```python
from build123d import *

# Parameters (mm, degrees)
SKETCH_W         = 45.6
SKETCH_H         = 44
SKETCH_R         = 2
PAD_DEPTH        = 3.5
PAD001_DEPTH     = 20
SKETCH002_W      = 3
SKETCH002_H      = 5
PAD002_DEPTH     = 1
CHAMFER_SIZE     = 1
CHAMFER001_ANGLE = 45
CHAMFER001_SIZE  = 2.5


with BuildPart() as part:
    # Sketch → Pad (new body)
    with BuildSketch(Plane.XY):
        Rectangle(SKETCH_W, SKETCH_H)
        with Locations((-11.4, 0)):
            Circle(SKETCH_R, mode=Mode.SUBTRACT)
        with Locations((11.4, 0)):
            Circle(SKETCH_R, mode=Mode.SUBTRACT)
    extrude(amount=PAD_DEPTH)

    # Sketch001 (on Face8 of Pad) → Pad001 (join)
    with BuildSketch(Plane.XY.offset(3.5)):
        Polygon((-22.8, 22), (-22.8, -22), (22.8, -22), (22.8, 22), (21.3, 22), (21.3, -20.5), (-21.3, -20.5), (-21.3, 22), align=None)
    extrude(amount=PAD001_DEPTH)

    # Sketch002 (on Face14 of Pad001) → Pad002 (join)
    with BuildSketch(Plane.XY.offset(23.5)):
        with Locations((-21.3, 19.5)):
            Rectangle(SKETCH002_W, SKETCH002_H)
        with Locations((21.3, 19.5)):
            Rectangle(SKETCH002_W, SKETCH002_H)
        with Locations((-21.3, -16.5)):
            Rectangle(SKETCH002_W, SKETCH002_H)
        with Locations((21.3, -16.5)):
            Rectangle(SKETCH002_W, SKETCH002_H)
    extrude(amount=PAD002_DEPTH)

    # Chamfer
    chamfer_edges = [part.edges().sort_by_distance(p)[0] for p in [
        (-21.3, -16.5, 23.5),
        (-21.3, 19.5, 23.5),
        (21.3, -16.5, 23.5),
        (21.3, 19.5, 23.5),
    ]]
    chamfer(chamfer_edges, length=CHAMFER_SIZE)

    # Chamfer001
    chamfer001_edges = [part.edges().sort_by_distance(p)[0] for p in [
        (9.4, 0, 3.5),
        (-13.4, 0, 3.5),
    ]]
    chamfer001_side = part.faces().sort_by_distance((0, 0.760558, 3.5))[0]
    chamfer(chamfer001_edges, length=CHAMFER001_SIZE, angle=CHAMFER001_ANGLE, reference=chamfer001_side)


solid = part.part
```
CAD build for the part. Positions are in the model's coordinates, mm. A direction names the side the tool comes from. Round coordinates to 2 decimals unless told otherwise and drop trailing zeros. Order: outer loops, then holes, each group sorted by start corner. A loop starts at its lowest first (then second) coordinate and runs counter-clockwise, first axis right, second up. Notation, with made-up numbers: (75.25, -24.75) - (134.25, -24.75) arc R28 ccw to (134.25, 8.25) - close; hole circle Ø1 at (49, -17). An arc over 180 degrees is marked (long way). Answer in a Markdown table with one row per item. Add a question column.
(1) Band-saw the part on A-A on y = 0. List the corners of the cut face in (x, z), and give its area (3 significant figures).
(2) Band-saw the part on D-D on y = -13. List the corners of the cut face in (x, z).
(3) Band-saw the part on B-B on x = -11.4. List the corners of the cut face in (y, z).
(4) 3-axis set-ups, long thin cutter, end or side, ignore diameter. For faces 4 (the face through (0, -21, 23.5)), 5 (the face through (22, 2, 23.5)), 6 (the face through (21, -19, 24)): which of +Z, -Z, +X, -X, +Y, -Y reach the whole face in a straight line?
(5) Mould opens along X. For faces 1 (the face through (-22.8, 0, 12)), 2 (the face through (-22, 2, 23.5)), 3 (the face through (21.3, 1, 13)) say: +X half, -X half, draft (parallel to the pull), parting line (faces both ways), or undercut.
(6) Probe L1, parallel to Y at x = 11.4, z = 0.7; L2, parallel to X at y = 0, z = 11.25; L3, parallel to Y at x = 3, z = 12.25. List the from-to ranges inside material, lowest first. Write a range as [from, to].
(7) Band-saw the part on C-C on z = 11. List the corners of the cut face in (x, y).
(8) Drop flat-ended pins along their axis: pin 1 Ø8 at (x, z) = (4, 12) entering from +Y; pin 2 Ø1.6 at (x, y) = (22.5, -3) entering from +Z; pin 3 Ø2.5 at (x, y) = (-11.4, 0) entering from +Z. Give the stop position or say it passes through.
Data:
| question | item | result |
|---|---|---|
| 1 | outline | (-22.8, 0) - (-13.4, 0) - (-13.4, 1) - (-15.9, 3.5) - (-21.3, 3.5) - (-21.3, 23.5) - (-22.8, 23.5) - close; (-9.4, 0) - (9.4, 0) - (9.4, 1) - (6.9, 3.5) - (-6.9, 3.5) - (-9.4, 1) - close; (13.4, 0) - (22.8, 0) - (22.8, 23.5) - (21.3, 23.5) - (21.3, 3.5) - (15.9, 3.5) - (13.4, 1) - close |
| 1 | area | 179 mm^2 |
| 2 | outline | (-22.8, 0) - (22.8, 0) - (22.8, 23.5) - (21.3, 23.5) - (21.3, 3.5) - (-21.3, 3.5) - (-21.3, 23.5) - (-22.8, 23.5) - close |
| 3 | outline | (-22, 0) - (-2, 0) - (-2, 1) - (-4.5, 3.5) - (-20.5, 3.5) - (-20.5, 23.5) - (-22, 23.5) - close; (2, 0) - (22, 0) - (22, 3.5) - (4.5, 3.5) - (2, 1) - close |
| 4 | face 4 | +Z, +X, -X, -Y |
| 4 | face 5 | +Z, +X, -X |
| 4 | face 6 | +Z |
| 5 | face 1 | -X half |
| 5 | face 2 | draft |
| 5 | face 3 | undercut |
| 6 | L1 | y = [-22, -2], [2, 22] |
| 6 | L2 | x = [-22.8, -21.3], [21.3, 22.8] |
| 6 | L3 | y = [-22, -20.5] |
| 7 | outline | (-22.8, -22) - (22.8, -22) - (22.8, 22) - (21.3, 22) - (21.3, -20.5) - (-21.3, -20.5) - (-21.3, 22) - (-22.8, 22) - close |
| 8 | pin 1 | stops at y = -20.5 |
| 8 | pin 2 | stops at z = 23.5 |
| 8 | pin 3 | passes through |
